from build123d import *

# Parameters (mm, degrees)
SKETCH2_W                    = 2347.722
SKETCH2_H                    = 63.5
BASE_FLANGE1_DEPTH           = 2.0574
EDGE_FLANGE1_STRIP_W         = 12.2936
EDGE_FLANGE1_STRIP_H         = 2.0574
EDGE_FLANGE1_STRIP_CUT_DEPTH = 2347.722
EDGE_FLANGE1_DEPTH           = 2347.722
EDGE_FLANGE1_FLAT_DEPTH      = 2.0574


# Sheet-metal steps are written as plain solids
with BuildPart() as part:
    # Sketch2 → Base-Flange1 (new body)
    with BuildSketch(Plane(origin=(0, 0, 0), x_dir=(1, 0, 0), z_dir=(0, 1, 0))):
        Rectangle(SKETCH2_W, SKETCH2_H)
    extrude(amount=-BASE_FLANGE1_DEPTH)

    # Edge-Flange1 strip (across the edge) → Edge-Flange1 strip cut (cut)
    with BuildSketch(Plane(origin=(-1173.861, -2.0574, -31.75), x_dir=(0, 0, 1), z_dir=(1, 0, 0))):
        with Locations((-2.0574, -1.0287)):
            Rectangle(EDGE_FLANGE1_STRIP_W, EDGE_FLANGE1_STRIP_H)
    edge_flange1_strip_cut = extrude(amount=EDGE_FLANGE1_STRIP_CUT_DEPTH, mode=Mode.SUBTRACT)

    # Edge-Flange1 bend section (across the edge) → Edge-Flange1 (add)
    with BuildSketch(Plane(origin=(-1173.861, -2.0574, -31.75), x_dir=(0, 0, 1), z_dir=(1, 0, 0))):
        with BuildLine():
            Line((0, 2.032), (2.0574, 2.032))
            ThreePointArc((2.0574, 2.032), (2.652559021, 0.595159021), (4.0894, 0))
            Line((4.0894, 0), (4.0894, -2.0574))
            ThreePointArc((4.0894, -2.0574), (1.197757529, -0.859642471), (0, 2.032))
        make_face()
    edge_flange1 = extrude(amount=EDGE_FLANGE1_DEPTH)

    # Edge-Flange1 profile (on flange) → Edge-Flange1 flat (add)
    with BuildSketch(Plane(origin=(0, -2.0574, -31.75), x_dir=(-1, 0, 0), z_dir=(0, 0, 1))):
        with BuildLine():
            Line((1176.401, 36.0426), (1176.401, 23.3426))
            Line((1176.401, 23.3426), (1173.861, 23.3426))
            Line((1173.861, 23.3426), (1173.861, 61.4426))
            Line((1173.861, 61.4426), (-1173.861, 61.4426))
            Line((-1173.861, 61.4426), (-1173.861, 23.3426))
            Line((-1173.861, 23.3426), (-1176.401, 23.3426))
            Line((-1176.401, 23.3426), (-1176.401, 36.0426))
            ThreePointArc((-1176.401, 36.0426), (-1179.576, 39.2176), (-1182.751, 36.0426))
            Line((-1182.751, 36.0426), (-1182.751, 15.24))
            Line((-1182.751, 15.24), (-1173.861, 6.35))
            Line((-1173.861, 6.35), (-1173.861, 2.032))
            Line((-1173.861, 2.032), (1173.861, 2.032))
            Line((1173.861, 2.032), (1173.861, 6.35))
            Line((1173.861, 6.35), (1182.751, 15.24))
            Line((1182.751, 15.24), (1182.751, 36.0426))
            ThreePointArc((1182.751, 36.0426), (1179.576, 39.2176), (1176.401, 36.0426))
        make_face()
    edge_flange1_flat = extrude(amount=EDGE_FLANGE1_FLAT_DEPTH)

    # Mirror1: Edge-Flange1 strip cut, Edge-Flange1, Edge-Flange1 flat across plane
    add(edge_flange1_strip_cut.mirror(Plane.XY), mode=Mode.SUBTRACT)
    add(edge_flange1.mirror(Plane.XY))
    add(edge_flange1_flat.mirror(Plane.XY))


solid = part.part
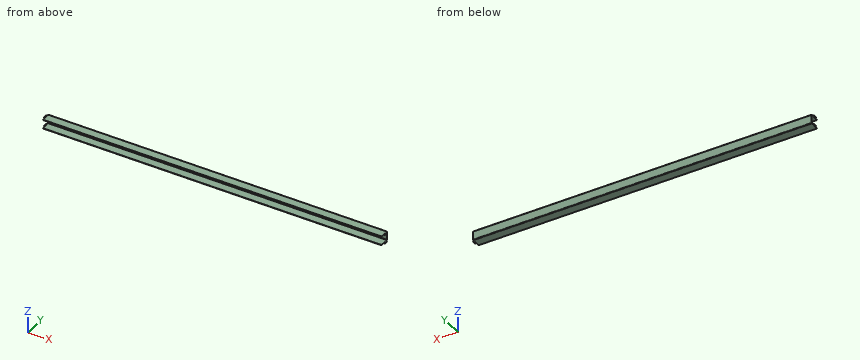
For this review, take the finished solid that the model builds, in its own axes (mm). Give positions to 0.01 mm unless a question says otherwise; leave off trailing zeros. Order: outer loops, then holes, each group sorted by start corner. A loop starts at its lowest first (then second) coordinate and runs counter-clockwise, first axis right, second up. Notation, with made-up numbers: (47, 9.25) -> (72, 9.25) arc R31 ccw to (72, 34.25) -> close; hole circle Ø11 at (85, 25). An arc over 180 degrees is marked (long way). Write item = value, one per line.
1) We need section A-A, the plane x = -174. Give the boundary of the cut face in (y, z).
Findings:
outline = (-63.5, -31.75) -> (-4.09, -31.75) arc R4.09 ccw to (0, -27.66) -> (0, 27.66) arc R4.09 ccw to (-4.09, 31.75) -> (-63.5, 31.75) -> (-63.5, 29.69) -> (-4.09, 29.69) arc R2.03 cw to (-2.06, 27.66) -> (-2.06, -27.66) arc R2.03 cw to (-4.09, -29.69) -> (-63.5, -29.69) -> close
2) Insertion check: pin 1 (4 mm diameter, centred on x = -18.5, z = 14.5, fed in from -Y); pin 2 (1.6 mm diameter, centred on y = -41.5, z = 30.5, fed in from -X); pin 3 (1 mm diameter, centred on x = 1175, z = 31, fed in from -Y); pin 4 (2.5 mm diameter, centred on y = -5, z = -8, fed in from -X). Each pin has a flat end and moves straight along its axis. Give the tip position at first contact, or say it passes through.
Findings:
pin_1 = -2.06
pin_2 = -1181.4
pin_3 = -25.4
pin_4 = through
3) To check wall thickness, follow L1, parallel to Z at x = 1000.5, y = -36; L2, parallel to Y at x = -595, z = 3.5. State the ranges of each line that lie inside material, in increasing order. Write a range as from..to.
Findings:
L1 = -31.75..-29.69, 29.69..31.75
L2 = -2.06..0
4) We need section B-B, the plane z = -16.5. Give the boundary of the cut face in (x, y), and give its area (3 significant figures).
Findings:
outline = (-1173.86, -2.06) -> (1173.86, -2.06) -> (1173.86, 0) -> (-1173.86, 0) -> close
area = 4,830 mm^2
